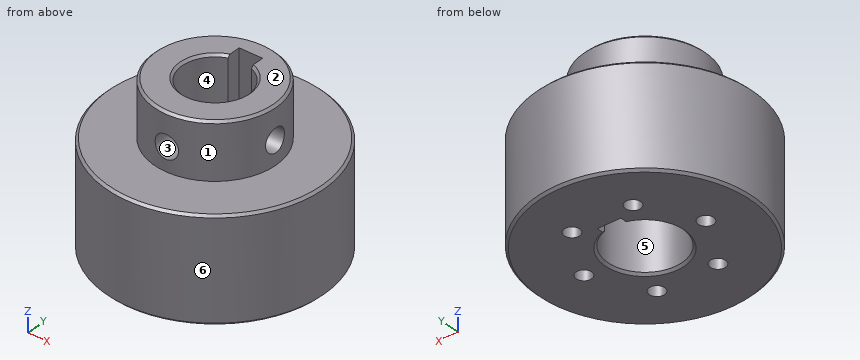
from build123d import *

# Parameters (mm, degrees)
SKETCH_1_R               = 23.2
SKETCH_1_R_2             = 7
EXTRUDE_1_DEPTH          = 34
SKETCH_2_R               = 34.674614003
SKETCH_2_R_2             = 13
CUT_EXTRUDE_1_DEPTH      = 12
HOLE_WIZARD_1_D          = 16
HOLE_WIZARD_1_DEPTH      = 15
SKETCH_3_W               = 5
SKETCH_3_H               = 10.2
CUT_EXTRUDE_2_DEPTH      = 48.249126976
SKETCH_4_W               = 2.5
SKETCH_4_H               = 23.2
PATTERN_CIRCULAR_2_COUNT = 6
PATTERN_CIRCULAR_1_COUNT = 2
PATTERN_CIRCULAR_1_ANGLE = 90
CHAMFER_1_SIZE           = 0.5


with BuildPart() as part:
    # 草图1 → 凸台-拉伸1 (new body)
    with BuildSketch(Plane.XY):
        Circle(SKETCH_1_R)
        Circle(SKETCH_1_R_2, mode=Mode.SUBTRACT)
    extrude(amount=EXTRUDE_1_DEPTH)

    # 草图2 → 切除-拉伸1 (cut)
    with BuildSketch(Plane.XY.offset(34)):
        Circle(SKETCH_2_R)
        Circle(SKETCH_2_R_2, mode=Mode.SUBTRACT)
    extrude(amount=-CUT_EXTRUDE_1_DEPTH, mode=Mode.SUBTRACT)

    # 孔1
    with Locations(Plane(origin=(0, 0, 0), x_dir=(-1, 0, 0), z_dir=(0, 0, -1))):
        with Locations((0, 0)):
            Hole(HOLE_WIZARD_1_D / 2, depth=HOLE_WIZARD_1_DEPTH)

    # 草图3 → 切除-拉伸2 (cut, through all)
    with BuildSketch(Plane.XY.offset(34)):
        with Locations((0, 4.4)):
            Rectangle(SKETCH_3_W, SKETCH_3_H)
    extrude(amount=-CUT_EXTRUDE_2_DEPTH, mode=Mode.SUBTRACT)

    # 草图4 → M6 螺纹孔1 (revolve, cut)
    with BuildSketch(Plane(origin=(0, 0, 27), x_dir=(0, 0, 1), z_dir=(1, 0, 0))):
        with Locations((1.25, 11.6)):
            Rectangle(SKETCH_4_W, SKETCH_4_H)
    hole_wizard_m6_1 = revolve(axis=Axis((0, 6.35, 27), (0, -1, 0)), mode=Mode.SUBTRACT)

    # 草图8 → M4 螺纹孔1 (revolve, cut)
    with BuildSketch(Plane.YZ.offset(-13)):
        Polygon((0, 0), (0, 11.091420021), (1.65, 10.1), (1.65, 0), align=None)
    hole_wizard_m4_1 = revolve(axis=Axis((-13, 0, -6.35), (0, 0, 1)), mode=Mode.SUBTRACT)

    # 阵列(圆周)2: M4 螺纹孔1 ×6 about axis
    pattern_circular_2_axis = Axis((0, 0, 0), (0, 0, 1))
    for i in range(1, PATTERN_CIRCULAR_2_COUNT):
        add(hole_wizard_m4_1.rotate(pattern_circular_2_axis, i * 360 / PATTERN_CIRCULAR_2_COUNT), mode=Mode.SUBTRACT)

    # 阵列(圆周)1: M6 螺纹孔1 ×2 about axis
    pattern_circular_1_axis = Axis((0, 0, 22), (0, 0, 1))
    for i in range(1, PATTERN_CIRCULAR_1_COUNT):
        add(hole_wizard_m6_1.rotate(pattern_circular_1_axis, i * PATTERN_CIRCULAR_1_ANGLE / (PATTERN_CIRCULAR_1_COUNT - 1)), mode=Mode.SUBTRACT)

    # 倒角1
    chamfer_1_edges = [part.edges().sort_by_distance(p)[0] for p in [
        (-23.2, 0, 22),
        (-13, 0, 34),
        (-23.2, 0, 0),
        (0, -8, 0),
        (0, -7, 34),
    ]]
    chamfer(chamfer_1_edges, length=CHAMFER_1_SIZE)


solid = part.part
Input: part model. Units: mm. Frame: model coordinates. Face numbers are marked on the shaded views. A direction names the side the tool comes from. Give positions to 0.01 mm unless a question says otherwise; leave off trailing zeros. Loops run counter-clockwise (first coordinate to the right, second up) from the corner with the lowest first, then second, coordinate; pieces in that order, holes last. Notation, with made-up numbers: (-31, -23) -> (-23, -23) arc R24 ccw to (-23, -5) -> close; hole circle Ø7 at (-34.5, -23.75). An arc over 180 degrees is marked (long way). Answer as a JSON object with one key per item and string values. Group by question number.
Item 1: Pin query (flat end, axial travel): P1, Ø6, axis at y = 0, z = 27, coming from the -X side; P2, Ø2.5, axis at y = 8.5, z = 18, coming from the -X side; P3, Ø2, axis at x = -6.5, y = -11.26, coming from the -Z side; P4, Ø2, axis at x = 4, y = 2, coming from the +Z side. Return the tip coordinate at first contact, or that it passes through.
Item 2: Cut plane B-B, the plane z = 27. Return the cut outline in (x, y).
Item 3: Line query: probe 1 along Z at (x, y) = (0, -10); probe 2 along X at (y, z) = (0, 7.5); probe 3 along X at (y, z) = (-0.5, 11). Output: solid intervals per line, ascending.
Item 4: Cut plane A-A, the plane z = 18.5. Return the cut outline in (x, y).
Item 5: Reachability of the marked faces 1 and 2 from +Z, -Z, +X, -X, +Y, -Y: full face, straight path, thin tool, end or side. Return the list, or none.
Item 6: Pull-direction query (Y, two-part tool) for the marked faces 3, 4, 5 and 6; classes: released by +Y, released by -Y, zero draft, split by the parting line, or undercut.
Checks:
{
 "1": {"P1": "stops at x = -13", "P2": "stops at x = -22.04", "P3": "stops at z = 10.49", "P4": "passes through"},
 "2": {"outline": "(-2.5, -12.76) -> (-2.5, -6.54) arc R7 cw to (-2.5, 6.54) -> (-2.5, 9.5) -> (2.5, 9.5) -> (2.5, 6.54) arc R7 cw to (6.54, 2.5) -> (12.76, 2.5) arc R13 ccw (long way) to start; (2.5, -12.76) arc R13 ccw to (12.76, -2.5) -> (6.54, -2.5) arc R7 cw to (2.5, -6.54) -> close"},
 "3": {"probe 1": "z = 0 to 24.5, 29.5 to 34", "probe 2": "x = -23.2 to -14.65, -11.35 to -8, 8 to 11.35, 14.65 to 23.2", "probe 3": "x = -23.19 to -7.98, 7.98 to 23.19"},
 "4": {"outline": "circle Ø46.4 at (0, 0); hole (-2.5, 6.54) arc R7 ccw (long way) to (2.5, 6.54) -> (2.5, 9.5) -> (-2.5, 9.5) -> close"},
 "5": {"face 1": "+Z", "face 2": "+Z, +X, -X, +Y, -Y"},
 "6": {"face 3": "zero draft", "face 4": "undercut", "face 5": "undercut", "face 6": "split by the parting line"}
}
